from build123d import *

# Parameters (mm, degrees)
SKETCH_1_R      = 4
EXTRUDE_1_DEPTH = 1


with BuildPart() as part:
    # 草圖1 → 填料-伸長1 (new body)
    with BuildSketch(Plane.XY):
        with BuildLine():
            Line((0, 21), (21, 21))
            Line((21, 21), (21, 0))
            Line((21, 0), (215, 0))
            ThreePointArc((215, 0), (219.242640687, 1.757359313), (221, 6))
            Line((221, 6), (221, 34.5))
            Line((221, 34.5), (227.535533906, 41.035533906))
            ThreePointArc((227.535533906, 41.035533906), (229.292893219, 45.278174593), (227.535533906, 49.52081528))
            Line((227.535533906, 49.52081528), (47.571067812, 229.485281374))
            ThreePointArc((47.571067812, 229.485281374), (43.328427125, 231.242640687), (39.085786438, 229.485281374))
            Line((39.085786438, 229.485281374), (30.600505063, 221))
            Line((30.600505063, 221), (0, 221))
            Line((0, 221), (0, 21))
        make_face()
        with Locations((10, 206)):
            Circle(SKETCH_1_R, mode=Mode.SUBTRACT)
        with Locations((10, 46)):
            Circle(SKETCH_1_R, mode=Mode.SUBTRACT)
        with Locations((10, 131)):
            Circle(SKETCH_1_R, mode=Mode.SUBTRACT)
        with Locations((46, 10)):
            Circle(SKETCH_1_R, mode=Mode.SUBTRACT)
        with Locations((131, 10)):
            Circle(SKETCH_1_R, mode=Mode.SUBTRACT)
        with Locations((206, 10)):
            Circle(SKETCH_1_R, mode=Mode.SUBTRACT)
    extrude(amount=EXTRUDE_1_DEPTH)


solid = part.part
Input: part model. Units: mm. Frame: model coordinates. Coordinates: 2 decimals unless noted, no trailing zeros. Loops run counter-clockwise (first coordinate to the right, second up) from the corner with the lowest first, then second, coordinate; pieces in that order, holes last. Notation, with made-up numbers: (-27, 66.25) -> (22, 66.25) arc R12 cw to (22, 73.25) -> close; hole circle Ø2 at (-12.5, 53). An arc over 180 degrees is marked (long way). Write item = value, one per line. Start each with the question number.
Item 1: Material intervals for line 1 (Y direction, x = 10, z = 0.55); line 2 (Y direction, x = 46, z = 0.35); line 3 (Y direction, x = 202.5, z = 0.8), sorted ascending.
Item 2: Cut plane A-A, the plane x = 10. Return loops of the section in (y, z), plus the area to 3 significant figures.
Item 3: Cut plane C-C, the plane z = 0.65. Return loops of the section in (x, y).
Item 4: First-contact query: P1, Ø9, axis at x = 131, y = 10, coming from the +Z side. Flat tip, straight axial feed; report the tip coordinate or a pass-through.
Item 5: Cut plane D-D, the plane x = 206. Return loops of the section in (y, z).
Item 6: Mould query, pull axis X, two halves, no side actions, for faces 1 (the face through (138.813, 138.243, 0.493)), 2 (the face through (42.004, 10.176, 0.493)), 3 (the face through (88, 92, 0)). Classes: pulls with the +X half, pulls with the -X half, needs draft (parallel to the pull), parting line crosses it, or undercut.
Ans:
q1.line_1 = 21 to 42, 50 to 127, 135 to 202, 210 to 221
q1.line_2 = 0 to 6, 14 to 230.62
q1.line_3 = 0 to 8.06, 11.94 to 74.56
q2.outline = (21, 0) -> (42, 0) -> (42, 1) -> (21, 1) -> close; (50, 0) -> (127, 0) -> (127, 1) -> (50, 1) -> close; (135, 0) -> (202, 0) -> (202, 1) -> (135, 1) -> close; (210, 0) -> (221, 0) -> (221, 1) -> (210, 1) -> close
q2.area = 176 mm²
q3.outline = (0, 21) -> (21, 21) -> (21, 0) -> (215, 0) arc R6 ccw to (221, 6) -> (221, 34.5) -> (227.54, 41.04) arc R6 ccw to (227.54, 49.52) -> (47.57, 229.49) arc R6 ccw to (39.09, 229.49) -> (30.6, 221) -> (0, 221) -> close; hole circle Ø8 at (10, 46); hole circle Ø8 at (10, 131); hole circle Ø8 at (10, 206); hole circle Ø8 at (46, 10); hole circle Ø8 at (131, 10); hole circle Ø8 at (206, 10)
q4.P1 = 1
q5.outline = (0, 0) -> (6, 0) -> (6, 1) -> (0, 1) -> close; (14, 0) -> (71.06, 0) -> (71.06, 1) -> (14, 1) -> close
q6.face_1 = pulls with the +X half
q6.face_2 = undercut
q6.face_3 = needs draft
